```python
from build123d import *

# Parameters (mm, degrees)
BOSS_EXTRUDE1_DEPTH = 3.175
SKETCH2_R           = 6.35
SKETCH2_R_2         = 1.5875
SKETCH2_R_3         = 2.032
CUT_EXTRUDE1_DEPTH  = 123.537765163
SKETCH3_R           = 2.032
SKETCH3_R_2         = 1.9685
CUT_EXTRUDE2_DEPTH  = 123.537765163
FILLET1_R           = 3.175
SKETCH4_R           = 2.032
CUT_EXTRUDE3_DEPTH  = 123.027997459
CUT_EXTRUDE4_REACH  = 124.028
FILLET2_R           = 1.5875


with BuildPart() as part:
    # Sketch1 → Boss-Extrude1 (new body)
    with BuildSketch(Plane.XY):
        with BuildLine():
            Line((102.692805421, 0), (-0.911395616, 0))
            Line((-0.911395616, 0), (-0.911395616, 25.4))
            Line((-0.911395616, 25.4), (-14.924855892, 25.4))
            Line((-14.924855892, 25.4), (-14.924855892, 63.605318816))
            ThreePointArc((-14.924855892, 63.605318816), (-13.994919922, 65.850382846), (-11.749855892, 66.780318816))
            Line((-11.749855892, 66.780318816), (35.462394108, 66.780318816))
            ThreePointArc((35.462394108, 66.780318816), (37.289381836, 66.201997626), (38.450803758, 64.677714623))
            Line((38.450803758, 64.677714623), (51.036631355, 29.605208386))
            ThreePointArc((51.036631355, 29.605208386), (53.359475199, 26.556642379), (57.013450653, 25.4))
            Line((57.013450653, 25.4), (98.214100111, 25.4))
            Line((98.214100111, 25.4), (102.692805421, 0))
        make_face()
    extrude(amount=BOSS_EXTRUDE1_DEPTH)

    # Sketch2 → Cut-Extrude1 (cut, through all)
    with BuildSketch(Plane.XY.offset(3.175)):
        with Locations((22.571894108, 50.206818816)):
            Circle(SKETCH2_R)
        with Locations((26.540644108, 16.5735)):
            Circle(SKETCH2_R)
        with Locations((-8.130355892, 30.5435)):
            Circle(SKETCH2_R_2)
        with Locations((35.811644108, 30.5435)):
            Circle(SKETCH2_R_2)
        with Locations((35.811644108, 2.6035)):
            Circle(SKETCH2_R_2)
        with Locations((-8.130355892, 2.6035)):
            Circle(SKETCH2_R_2)
        with Locations((-12.099105892, 36.236818816)):
            Circle(SKETCH2_R_2)
        with Locations((31.842894108, 36.236818816)):
            Circle(SKETCH2_R_2)
        with Locations((31.842894108, 64.176818816)):
            Circle(SKETCH2_R_2)
        with Locations((-12.099105892, 64.176818816)):
            Circle(SKETCH2_R_2)
        with Locations((66.180305421, 7.14375)):
            Circle(SKETCH2_R_3)
    extrude(amount=-CUT_EXTRUDE1_DEPTH, mode=Mode.SUBTRACT)

    # Sketch3 → Cut-Extrude2 (cut, through all)
    with BuildSketch(Plane(origin=(0, 0, 0), x_dir=(-1, 0, 0), z_dir=(0, 0, -1))):
        with Locations((-42.489558108, 39.189568816)):
            Circle(SKETCH3_R)
        with Locations((-4.644854384, 19.05)):
            Circle(SKETCH3_R_2)
        with Locations((-4.644854384, 6.35)):
            Circle(SKETCH3_R_2)
    extrude(amount=-CUT_EXTRUDE2_DEPTH, mode=Mode.SUBTRACT)

    # Fillet1
    fillet1_edges = [part.edges().sort_by_distance(p)[0] for p in [
        (-14.924855892, 25.4, 1.5875),
        (98.214100111, 25.4, 1.5875),
        (102.692805421, 0, 1.5875),
        (-0.911395616, 0, 1.5875),
    ]]
    fillet(fillet1_edges, radius=FILLET1_R)

    # Sketch4 → Cut-Extrude3 (cut, through all)
    with BuildSketch(Plane.XY.offset(3.175)):
        with Locations((94.755305421, 19.05)):
            Circle(SKETCH4_R)
        with Locations((97.126377465, 6.35)):
            Circle(SKETCH4_R)
        with Locations((-2.224855892, 60.430318816)):
            Circle(SKETCH4_R)
        with Locations((-2.224855892, 31.855318816)):
            Circle(SKETCH4_R)
    extrude(amount=-CUT_EXTRUDE3_DEPTH, mode=Mode.SUBTRACT)

    # Sketch5 → Cut-Extrude4 (cut, up to next)
    with BuildSketch(Plane(origin=(0, 0, 0), x_dir=(-1, 0, 0), z_dir=(0, 0, -1)), mode=Mode.PRIVATE) as cut_extrude4_sk1:
        Polygon((-3.064970502, 55.667818816), (-26.831361929, 32.965995206), (-16.361313511, 22.004969641), (3.812355892, 41.275), (8.574855892, 41.275), (8.574855892, 55.667818816), align=None)
    cut_extrude4_tool1 = extrude(cut_extrude4_sk1.sketch, amount=-CUT_EXTRUDE4_REACH, mode=Mode.PRIVATE) & part.part
    # Sketch5 → Cut-Extrude4 (cut, up to next)
    with BuildSketch(Plane(origin=(0, 0, 0), x_dir=(-1, 0, 0), z_dir=(0, 0, -1)), mode=Mode.PRIVATE) as cut_extrude4_sk2:
        Polygon((-92.270683803, 4.2545), (-89.29642955, 21.122334072), (-70.24642955, 21.122334072), (-73.220683803, 4.2545), align=None)
    cut_extrude4_tool2 = extrude(cut_extrude4_sk2.sketch, amount=-CUT_EXTRUDE4_REACH, mode=Mode.PRIVATE) & part.part
    # Sketch5 → Cut-Extrude4 (cut, up to next)
    with BuildSketch(Plane(origin=(0, 0, 0), x_dir=(-1, 0, 0), z_dir=(0, 0, -1)), mode=Mode.PRIVATE) as cut_extrude4_sk3:
        Polygon((-40.089927038, 4.2545), (-59.139927038, 4.2545), (-62.114181291, 21.122334072), (-43.064181291, 21.122334072), align=None)
    cut_extrude4_tool3 = extrude(cut_extrude4_sk3.sketch, amount=-CUT_EXTRUDE4_REACH, mode=Mode.PRIVATE) & part.part
    add(cut_extrude4_tool1.solids().sort_by_distance((7.67675, 40.461869, 0))[0], mode=Mode.SUBTRACT)
    add(cut_extrude4_tool2.solids().sort_by_distance((81.258557, 12.688417, 0))[0], mode=Mode.SUBTRACT)
    add(cut_extrude4_tool3.solids().sort_by_distance((51.102054, 12.688417, 0))[0], mode=Mode.SUBTRACT)

    # Fillet2
    fillet2_edges = [part.edges().sort_by_distance(p)[0] for p in [
        (3.064970502, 55.667818816, 1.5875),
        (-8.574855892, 55.667818816, 1.5875),
        (-8.574855892, 41.275, 1.5875),
        (-3.812355892, 41.275, 1.5875),
        (16.361313511, 22.004969641, 1.5875),
        (26.831361929, 32.965995206, 1.5875),
        (73.220683803, 4.2545, 1.5875),
        (92.270683803, 4.2545, 1.5875),
        (89.29642955, 21.122334072, 1.5875),
        (70.24642955, 21.122334072, 1.5875),
        (43.064181291, 21.122334072, 1.5875),
        (40.089927038, 4.2545, 1.5875),
        (59.139927038, 4.2545, 1.5875),
        (62.114181291, 21.122334072, 1.5875),
    ]]
    fillet(fillet2_edges, radius=FILLET2_R)


solid = part.part
```
Here's how the part is built. I have some questions about the finished solid (model axes, mm). A direction names the side the tool comes from. Round coordinates to 2 decimals unless told otherwise and drop trailing zeros. Write each loop counter-clockwise with the first axis right and the second up, starting at its lowest first coordinate (ties: lowest second). Pieces come first, ordered by that corner, then holes.
Q1. Please list where these lines run through material, in increasing order: probe 1 along Y at (x, z) = (79, 0.65); probe 2 along X at (y, z) = (35, 1.2); probe 3 along X at (y, z) = (16.5, 0.9).
Q2. Will these pins go through, and if not, where does the flat tip stop? P1, Ø20.5, axis at x = 22.57, y = 50.21, coming from the +Z side (3 decimals); P2, Ø3, axis at x = -12.1, y = 36.24, coming from the +Z side; P3, Ø1.6, axis at x = -1, z = 1, coming from the -Y side.
Q3. Which directions (+Z, -Z, +X, -X, +Y, -Y) give clear straight access to the entire face, cutting with the end or side of a thin tool? Please do faces 5 (the flat face through (76, 25.4, 2)), 6 (the flat face through (-6, 41.275, 2)).
Q4. If we section it at A-A on x = 84: Write out the boundary of the cut face in (y, z) (1 decimal).
Q5. If we section it at C-C on z = 2.5: Give the number of separate pieces and of enclosed holes in the cut face, plus the area to 3 significant figures.
Q6. If we section it at D-D on x = 48: Write out the boundary of the cut face in (y, z) (1 decimal), plus the area to 3 significant figures.
Q7. If we mould it in two halves opening along Y, with no side actions, what happens to faces 1 (the cylindrical face through (31.64, 65.75, 1.61)), 2 (the flat face through (14.45, 44.79, 1.57)), 3 (the flat face through (-6, 25.4, 2)), 4 (the flat face through (31, 26, 3.175))? For each: +Y half, -Y half, draft (parallel to the pull), parting line (faces both ways), or undercut.
Q8. If we section it at B-B on y = 12: Write out the boundary of the cut face in (x, z) (3 decimals).
Answer below:
1. probe 1: y = 0 to 4.25, 21.12 to 25.4
1. probe 2: x = -14.92 to -13.09, -11.1 to 2.76, 24.7 to 30.85, 32.84 to 49.1
1. probe 3: x = -0.91 to 20.19, 32.89 to 42.25, 61.3 to 71.06, 90.11 to 99.78
2. P1: stops at z = 3.175
2. P2: passes through
2. P3: stops at y = 1.17
3. face 5: +Z, -Z, +X, +Y
3. face 6: +Z, -Z
4. outline: (0, 0) - (4.3, 0) - (4.3, 3.2) - (0, 3.2) - close; (21.1, 0) - (25.4, 0) - (25.4, 3.2) - (21.1, 3.2) - close
5. separate pieces: 1
5. enclosed holes: 20
5. area: 3,430 mm2
6. outline: (0, 0) - (4.3, 0) - (4.3, 3.2) - (0, 3.2) - close; (21.1, 0) - (38.1, 0) - (38.1, 3.2) - (21.1, 3.2) - close
6. area: 67.3 mm2
7. face 1: undercut
7. face 2: undercut
7. face 3: -Y half
7. face 4: draft
8. outline: (-0.911, 0) - (22.135, 0) - (22.135, 3.175) - (-0.911, 3.175) - close; (30.946, 0) - (41.456, 0) - (41.456, 3.175) - (30.946, 3.175) - close; (60.506, 0) - (71.855, 0) - (71.855, 3.175) - (60.506, 3.175) - close; (90.905, 0) - (100.577, 0) - (100.577, 3.175) - (90.905, 3.175) - close
